Design review of the part built by this model. Coordinates are the model's own, in mm. A direction names the side the tool comes from. Round coordinates to 2 decimals unless told otherwise and drop trailing zeros. Loops run counter-clockwise (first coordinate to the right, second up) from the corner with the lowest first, then second, coordinate; pieces in that order, holes last. Notation, with made-up numbers: (78.25, -15.75) -> (116.25, -15.75) arc R15 cw to (116.25, -3.75) -> close; hole circle Ø2 at (-16.75, 10.5). An arc over 180 degrees is marked (long way). Use a Markdown table: item, result. Add a question column.
from build123d import *

# Parameters (mm, degrees)
F6_DEPTH = 12.5
F0_R     = 21.9
F0_R_2   = 28.15
F1_DEPTH = 31.25
F2_DEPTH = 5
F4_DEPTH = 130.647779
F5_R     = 5


with BuildPart() as f6:
    # F0 (on Top) → F6 (new body)
    with BuildSketch(Plane.XY):
        with BuildLine():
            ThreePointArc((-78.54655, 56.201151), (-40.29536, 38.937299), (-24.6403, 0))
            ThreePointArc((-24.6403, 0), (-40.29536, -38.937299), (-78.54655, -56.201151))
            Line((-78.54655, -56.201151), (220.932616, -43.712006))
            ThreePointArc((220.932616, -43.712006), (175.3597, 0), (220.932616, 43.712006))
            Line((220.932616, 43.712006), (-78.54655, 56.201151))
        make_face()
    extrude(amount=F6_DEPTH)

    # F0 (on Top) → F1 (join)
    with BuildSketch(Plane.XY):
        with BuildLine():
            ThreePointArc((262.8597, 0), (250.683543, 30.284566), (220.932616, 43.712006))
            ThreePointArc((220.932616, 43.712006), (175.3597, 0), (220.932616, -43.712006))
            ThreePointArc((220.932616, -43.712006), (250.683543, -30.284566), (262.8597, 0))
        make_face()
        with Locations((219.1097, 0)):
            Circle(F0_R, mode=Mode.SUBTRACT)
        with BuildLine():
            ThreePointArc((-78.54655, -56.201151), (-40.29536, -38.937299), (-24.6403, 0))
            ThreePointArc((-24.6403, 0), (-40.29536, 38.937299), (-78.54655, 56.201151))
            ThreePointArc((-78.54655, 56.201151), (-137.1403, 0), (-78.54655, -56.201151))
        make_face()
        with Locations((-80.8903, 0)):
            Circle(F0_R_2, mode=Mode.SUBTRACT)
    extrude(amount=F1_DEPTH)

    # F7 (on face) → F2 (cut)
    with BuildSketch(Plane.XY.offset(12.5)):
        with BuildLine():
            ThreePointArc((159.013575, -21.272479), (155.3597, 0), (159.013575, 21.272479))
            Line((159.013575, 21.272479), (-10.09648, 28.324856))
            ThreePointArc((-10.09648, 28.324856), (-4.6403, 0), (-10.09648, -28.324856))
            Line((-10.09648, -28.324856), (159.013575, -21.272479))
        make_face()
    extrude(amount=-F2_DEPTH, mode=Mode.SUBTRACT)

    # F3 (on face) → F4 (cut)
    with BuildSketch(Plane.XY.offset(31.25)):
        Polygon((-44.3303, 6.3), (-80.8903, 6.3), (-80.8903, 0), (-80.8903, -6.3), (-44.3303, -6.3), (-44.3303, 0), align=None)
    extrude(amount=-F4_DEPTH, mode=Mode.SUBTRACT)

    # F5
    f5_edges = [f6.edges().sort_by_distance(p)[0] for p in [
        (-83.23405, 56.201151, 31.25),
        (217.286783, 43.712006, 31.25),
    ]]
    fillet(f5_edges, radius=F5_R)

    # F8: F6 across face


with BuildPart() as f6_1:
    add(f6.part)
    add(f6.part.mirror(Plane(origin=(57.759203, 0, 0), x_dir=(1, 0, 0), z_dir=(0, 0, -1))))


solid = f6_1.part
1. Insertion check: P1, Ø17, axis at x = 67, y = 5, coming from the +Z side; P2, Ø2, axis at y = 17.5, z = 5.5, coming from the +X side; P3, Ø17, axis at x = 67.5, y = -9, coming from the -Z side. Each pin has a flat end and moves straight along its axis. Give the tip position at first contact, or say it passes through.
2. Consider section C-C on x = 43.5. State the section outline as (y, z) points, plus the area to 3 significant figures.
3. Mouldability with a two-part tool opening along X and no side actions: class faces 6 (the face through (236, -17, 31.25)), 7 (the face through (73.29, 49.87, 0.18)), 8 (the face through (-49, -6.3, 0)) as +X half, -X half, draft (parallel to the pull), parting line (faces both ways), or undercut.
4. For faces 1 (the face through (-59, -22, 31.25)), 2 (the face through (75.64, 24.75, 10.04)), 3 (the face through (236, -17, -31.25)), 4 (the face through (-49, 6.3, 0)), 5 (the face through (73, 0, -7.5)), list the 3-axis set-ups (+Z, -Z, +X, -X, +Y, -Y) from which the entire face can be reached by the end or side of a thin tool; tool diameter is ignored.
5. Consider section A-A on z = 3.5. State the section outline as (x, y) points, plus the area to 3 significant figures.
6. Consider section B-B on x = 105. State the section outline as (y, z) points (3 decimals), plus the area to 3 significant figures.
7. To check wall thickness, follow probe 1 along X at (y, z) = (19, -0.5); probe 2 along X at (y, z) = (-10, -26); probe 3 along X at (y, z) = (-25, 18). State the ranges of each line that lie inside material, in increasing order. Write a range as from..to.
Verdict:
| question | item | result |
|---|---|---|
| 1 | P1 | stops at z = 7.5 |
| 1 | P2 | stops at x = 259.63 |
| 1 | P3 | stops at z = -7.5 |
| 2 | outline | (-51.11, -12.5) -> (-26.09, -12.5) -> (-26.09, -7.5) -> (26.09, -7.5) -> (26.09, -12.5) -> (51.11, -12.5) -> (51.11, 12.5) -> (26.09, 12.5) -> (26.09, 7.5) -> (-26.09, 7.5) -> (-26.09, 12.5) -> (-51.11, 12.5) -> close |
| 2 | area | 2,030 mm² |
| 3 | face 6 | draft |
| 3 | face 7 | +X half |
| 3 | face 8 | undercut |
| 4 | face 1 | +Z, +X, -X, +Y, -Y |
| 4 | face 2 | +Z |
| 4 | face 3 | -Z, +X, -X, +Y, -Y |
| 4 | face 4 | +Z, -Z |
| 4 | face 5 | -Z |
| 5 | outline | (-78.55, -56.2) -> (220.93, -43.71) arc R43.75 ccw to (220.93, 43.71) -> (-78.55, 56.2) arc R56.25 ccw (long way) to start; hole (-53.45, -6.3) -> (-44.33, -6.3) -> (-44.33, 6.3) -> (-53.45, 6.3) arc R28.15 ccw (long way) to start; hole circle Ø43.8 at (219.11, 0) |
| 5 | area | 33,900 mm² |
| 6 | outline | (-48.547, -12.5) -> (-23.525, -12.5) -> (-23.525, -7.5) -> (23.525, -7.5) -> (23.525, -12.5) -> (48.547, -12.5) -> (48.547, 12.5) -> (23.525, 12.5) -> (23.525, 7.5) -> (-23.525, 7.5) -> (-23.525, 12.5) -> (-48.547, 12.5) -> close |
| 6 | area | 1,960 mm² |
| 7 | probe 1 | x = -133.83..-101.66, -60.12..208.22, 230..258.52 |
| 7 | probe 2 | x = -136.24..-107.2, -54.58..-25.54, 176.52..199.63, 238.59..261.7 |
| 7 | probe 3 | x = -131.28..-93.83, -67.95..-30.5, 183.21..255.01 |
